```python
from build123d import *

# Parameters (mm, degrees)
BOSS_EXTRUDE1_DEPTH = 10
FILLET1_START       = -1
FILLET1_DEPTH       = 12
FILLET1_2_DEPTH     = 10
FILLET2_R           = 1
FILLET3_R           = 0.25
SKETCH2_R           = 2
CUT_EXTRUDE1_DEPTH  = 26.785330572


with BuildPart() as part:
    # Sketch1 → Boss-Extrude1 (new body)
    with BuildSketch(Plane(origin=(0, 0, 0), x_dir=(0, 0, -1), z_dir=(1, 0, 0))):
        with BuildLine():
            Line((0, 0), (0, 8))
            Line((0, 8), (10, 8))
            Line((10, 8), (10, 6))
            Line((10, 6), (12, 6))
            ThreePointArc((12, 6), (17.480620462, 7.92151485), (22.5, 5))
            Line((22.5, 5), (20.689313396, 4))
            ThreePointArc((20.689313396, 4), (14.863284967, 5.218025808), (12, 0))
            Line((12, 0), (11, 0))
            ThreePointArc((11, 0), (9, 2), (7, 0))
            Line((7, 0), (5, 0))
            ThreePointArc((5, 0), (3, 2), (1, 0))
            Line((1, 0), (0, 0))
        make_face()
    extrude(amount=BOSS_EXTRUDE1_DEPTH)

    # Fillet1: read off the stored shape, not the designer's step
    # Fillet1 outline → Fillet1 (cut)
    with BuildSketch(Plane.YZ.offset(FILLET1_START)):
        with BuildLine():
            ThreePointArc((6, 0), (7.414213562, -0.585786438), (8, -2))
            Line((8, -2), (8, 0))
            Line((8, 0), (6, 0))
        make_face()
    extrude(amount=FILLET1_DEPTH, mode=Mode.SUBTRACT)

    # Fillet1 2 outline → Fillet1 2 (add)
    with BuildSketch(Plane.YZ):
        with BuildLine():
            ThreePointArc((6, -12), (6.585786438, -10.585786438), (8, -10))
            Line((8, -10), (6, -10))
            Line((6, -10), (6, -12))
        make_face()
    extrude(amount=FILLET1_2_DEPTH)

    # Fillet2
    fillet2_edges = [part.edges().sort_by_distance(p)[0] for p in [
        (5, 6, -12),
    ]]
    fillet(fillet2_edges, radius=FILLET2_R)

    # Fillet3
    fillet3_edges = [part.edges().sort_by_distance(p)[0] for p in [
        (5, 0, 0),
        (5, 5, -22.5),
        (5, 4, -20.689313396),
        (5, 0, -12),
        (5, 0, -11),
        (5, 0, -7),
        (5, 0, -5),
        (5, 0, -1),
    ]]
    fillet(fillet3_edges, radius=FILLET3_R)

    # Sketch2 → Cut-Extrude1 (cut, through all)
    with BuildSketch(Plane(origin=(0, 8, 0), x_dir=(1, 0, 0), z_dir=(0, 1, 0))):
        with Locations(Location((5, 8, 0), (0, 0, 321.827292373))):
            Circle(SKETCH2_R)
    extrude(amount=-CUT_EXTRUDE1_DEPTH, mode=Mode.SUBTRACT)


solid = part.part
```
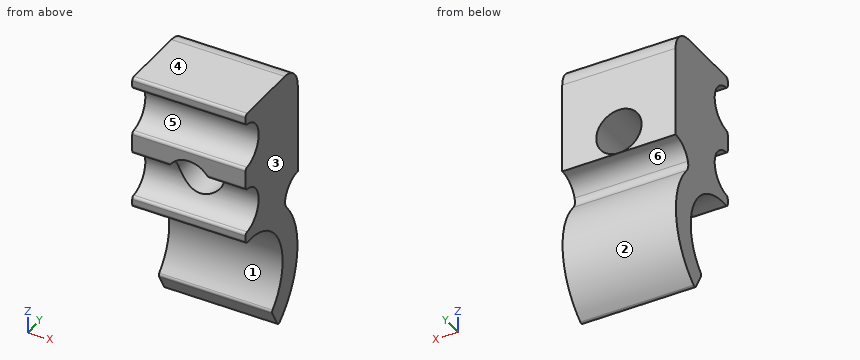
Work out the finished part from the listing and answer in its coordinate system (mm). Face numbers are marked on the shaded views. A direction names the side the tool comes from. Give positions to 0.01 mm unless a question says otherwise; leave off trailing zeros. Order: outer loops, then holes, each group sorted by start corner. A loop starts at its lowest first (then second) coordinate and runs counter-clockwise, first axis right, second up. Notation, with made-up numbers: (24, 73) -> (35, 73) arc R13 ccw to (35, 83) -> close; hole circle Ø3 at (63, 31.25). An arc over 180 degrees is marked (long way). Answer as CSV lines item,"result". Start each with the question number.
(1) Section B-B, the plane z = -8 is taken. Write down the section's boundary in (x, y), plus the area to 3 significant figures.
(2) Consider line 1 along X through (y, z) = (4, -8); line 2 along Z through (x, y) = (5, 2.75); line 3 along X through (y, z) = (5, -7.5). Determine where each line is inside the solid, lowest interval first.
(3) For a pull along Z with two mould halves and no side action, classify the marked faces 1, 2, 3 and 4 as released by +Z, released by -Z, zero draft, split by the parting line, or undercut.
(4) Section A-A, the plane y = 1.75 is taken. Write down the section's boundary in (x, z).
(5) Section C-C, the plane y = 3.75 is taken. Write down the section's boundary in (x, z).
(6) This flat-tipped pin is pushed along its axis until it touches: pin 1 Ø3 at (x, z) = (5, -8) entering from +Y. Where does it stop, or does it pass through?
(7) Which of the six approach directions +Z, -Z, +X, -X, +Y, -Y give full straight-line access (tool end or side, diameter ignored) to the marked faces 5 and 6?
Entries:
1,outline,"(0, 1.73) -> (3, 1.73) -> (3, 8) -> (0, 8) -> close; (7, 1.73) -> (10, 1.73) -> (10, 8) -> (7, 8) -> close"
1,area,"37.6 mm²"
2,line 1,"0 to 3, 7 to 10"
2,line 2,"-12.4 to -10, -6 to 0"
2,line 3,"0 to 3.06, 6.94 to 10"
3,face 1,"undercut"
3,face 2,"undercut"
3,face 3,"zero draft"
3,face 4,"released by +Z"
4,outline,"(0, -12.07) -> (10, -12.07) -> (10, -9.97) -> (5.35, -9.97) arc R2 cw to (4.65, -9.97) -> (0, -9.97) -> close; (0, -8.03) -> (3, -8.03) arc R2 cw (long way) to (7, -8.03) -> (10, -8.03) -> (10, -3.97) -> (0, -3.97) -> close; (0, -2.03) -> (10, -2.03) -> (10, 0) -> (0, 0) -> close"
5,outline,"(0, -13.01) -> (10, -13.01) -> (10, 0) -> (0, 0) -> close; hole circle Ø4 at (5, -8)"
6,pin 1,"through"
7,face 5,"+X, -X, -Y"
7,face 6,"+X, -X, +Y"
